Source: three-view drawing plus pictorial views. Frame: mm from the lowest corner of the part. Round coordinates to 2 decimals unless told otherwise and drop trailing zeros. Write each loop counter-clockwise with the first axis right and the second up, starting at its lowest first coordinate (ties: lowest second). Pieces come first, ordered by that corner, then holes. Notation, with made-up numbers: M 19,-28.5 L 67,-28.5 A26 ccw 67,-11.5 Z; hole C 66,79.5 d5. An arc over 180 degrees is marked long. Put each result on its own line as item: value. Start each with the question number.
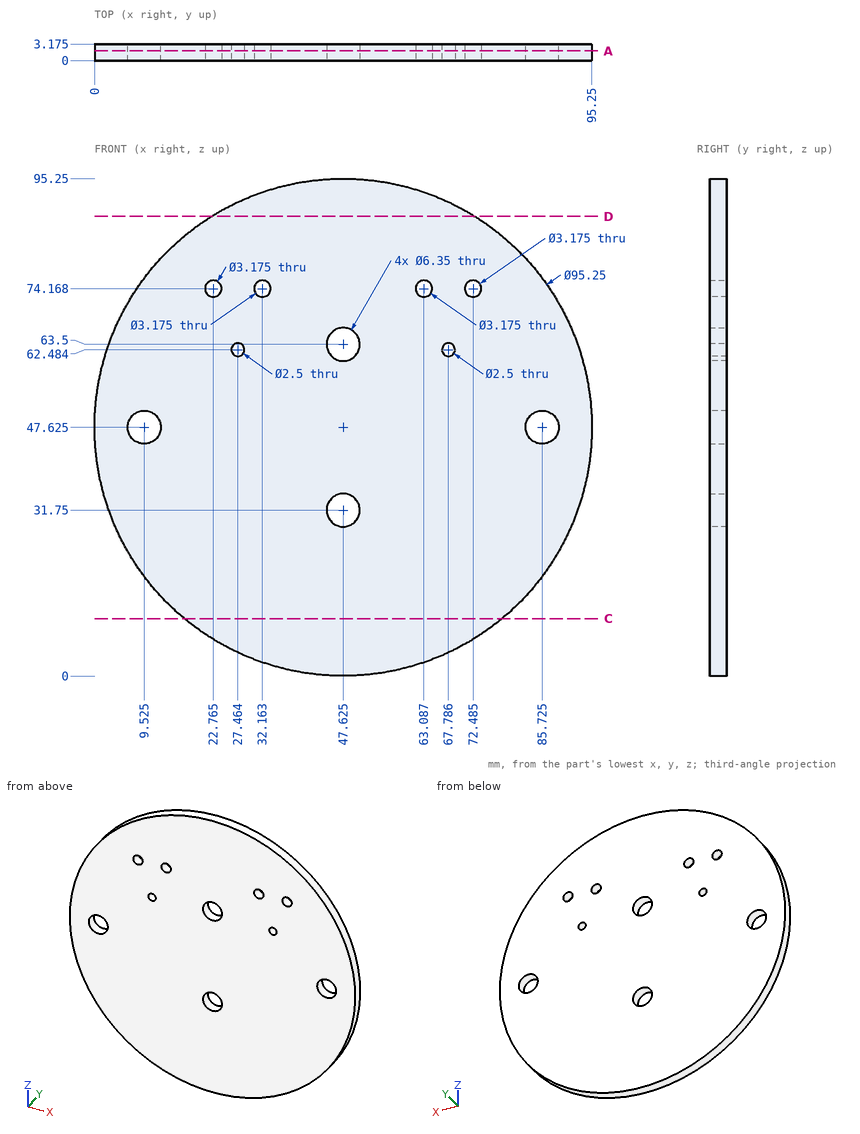
(1) Ray query, line 1 along X through (y, z) = (1.7, 34.5) (1 decimal); line 2 along X through (y, z) = (0.6, 31.5); line 3 along Z through (x, y) = (71.5, 0.6). Return the intervals inside material, ascending.
(2) Section query C-C (z = 11). Return loops of the section in (x, y) (1 decimal), and give its area (3 significant figures).
(3) Section query A-A (y = 1.85). Count the separate pieces of the cut face and the enclosed holes in it, and give its area (3 significant figures).
(4) Contact query for a flat-ended pin moving along its axis: P1, Ø4, axis at x = 47.625, z = 31.75, coming from the +Y side. Output: stop coordinate, or through.
(5) Section query D-D (z = 88). Return loops of the section in (x, y) (1 decimal), and give its area (3 significant figures).
Entries:
1. line 1: 1.8 to 46, 49.2 to 93.4
1. line 2: 2.81 to 44.46, 50.79 to 92.44
1. line 3: 6.42 to 72.92, 75.41 to 88.83
2. outline: M 17.2,0 L 78.1,0 L 78.1,3.2 L 17.2,3.2 Z
2. area: 193 mm2
3. separate pieces: 1
3. enclosed holes: 10
3. area: 6,960 mm2
4. P1: through
5. outline: M 22.4,0 L 72.9,0 L 72.9,3.2 L 22.4,3.2 Z
5. area: 160 mm2
